```python
from build123d import *

# Parameters (mm, degrees)
SKETCH1_R           = 4.5
SKETCH1_R_2         = 5
BOSS_EXTRUDE2_DEPTH = 3


with BuildPart() as part:
    # Sketch1 → Boss-Extrude2 (new body)
    with BuildSketch(Plane.XY):
        with BuildLine():
            Line((400, 6), (0, 6))
            ThreePointArc((0, 6), (-6, 0), (0, -6))
            Line((0, -6), (95, -6))
            Line((95, -6), (95, -35))
            ThreePointArc((95, -35), (100, -40), (105, -35))
            Line((105, -35), (105, -6))
            Line((105, -6), (155, -6))
            Line((155, -6), (155, -35))
            ThreePointArc((155, -35), (160, -40), (165, -35))
            Line((165, -35), (165, -6))
            Line((165, -6), (215, -6))
            Line((215, -6), (215, -35))
            ThreePointArc((215, -35), (220, -40), (225, -35))
            Line((225, -35), (225, -6))
            Line((225, -6), (275, -6))
            Line((275, -6), (275, -35))
            ThreePointArc((275, -35), (280, -40), (285, -35))
            Line((285, -35), (285, -6))
            Line((285, -6), (400, -6))
            ThreePointArc((400, -6), (406, 0), (400, 6))
        make_face()
        Circle(SKETCH1_R, mode=Mode.SUBTRACT)
        with Locations((400, 0)):
            Circle(SKETCH1_R_2, mode=Mode.SUBTRACT)
        with Locations((100, -35)):
            Circle(SKETCH1_R, mode=Mode.SUBTRACT)
        with Locations((280, -35)):
            Circle(SKETCH1_R, mode=Mode.SUBTRACT)
        with Locations((160, -35)):
            Circle(SKETCH1_R, mode=Mode.SUBTRACT)
        with Locations((220, -35)):
            Circle(SKETCH1_R, mode=Mode.SUBTRACT)
    extrude(amount=BOSS_EXTRUDE2_DEPTH)


solid = part.part
```
Work out the finished part from the listing and answer in its coordinate system (mm). Coordinates: 2 decimals unless noted, no trailing zeros. Order: outer loops, then holes, each group sorted by start corner. A loop starts at its lowest first (then second) coordinate and runs counter-clockwise, first axis right, second up. Notation, with made-up numbers: M 13.5,-11 L 41.5,-11 A19 cw 41.5,6 Z; hole C 83,36.5 d8. An arc over 180 degrees is marked long. Use CSV: the item, a comma, the result in double quotes.
1) Consider line 1 (X direction, y = -23, z = 1.25); line 2 (Y direction, x = 160, z = 1.8); line 3 (Y direction, x = 400, z = 0.85). Determine where each line is inside the solid, lowest interval first. Write a range as [from, to].
Worked out:
line 1,"x = [95, 105], [155, 165], [215, 225], [275, 285]"
line 2,"y = [-40, -39.5], [-30.5, 6]"
line 3,"y = [-6, -5], [5, 6]"
2) Section D-D on x = 100 is taken. Write down the section's boundary in (y, z).
Worked out:
outline,"M -40,0 L -39.5,0 L -39.5,3 L -40,3 Z; M -30.5,0 L 6,0 L 6,3 L -30.5,3 Z"
3) Section A-A on y = -19.5 is taken. Write down the section's boundary in (x, z).
Worked out:
outline,"M 95,0 L 105,0 L 105,3 L 95,3 Z; M 155,0 L 165,0 L 165,3 L 155,3 Z; M 215,0 L 225,0 L 225,3 L 215,3 Z; M 275,0 L 285,0 L 285,3 L 275,3 Z"
4) Section B-B on y = 0 is taken. Write down the section's boundary in (x, z).
Worked out:
outline,"M -6,0 L -4.5,0 L -4.5,3 L -6,3 Z; M 4.5,0 L 395,0 L 395,3 L 4.5,3 Z; M 405,0 L 406,0 L 406,3 L 405,3 Z"
5) Flat-ended cylindrical pins translate along their axes: pin 1 Ø1.5 at (y, z) = (-18.5, 2) entering from -X; pin 2 Ø1.5 at (y, z) = (-17.5, 1.5) entering from +X; pin 3 Ø1.5 at (x, z) = (65, 2) entering from -Y. Find the tip coordinate at first contact, or state that the pin passes through.
Worked out:
pin 1,"stops at x = 95"
pin 2,"stops at x = 285"
pin 3,"stops at y = -6"
6) Determine the mould class of faces 1 (the face through (224.16, -36.72, 1.48)), 2 (the face through (-0.59, 4.46, 1.48)), 3 (the face through (199, -2, 0)) for opening direction X: released by +X, released by -X, zero draft, split by the parting line, or undercut.
Worked out:
face 1,"undercut"
face 2,"undercut"
face 3,"zero draft"
7) Section C-C on z = 1.1 is taken. Write down the section's boundary in (x, y), plus the area to 3 significant figures.
Worked out:
outline,"M 0,-6 L 95,-6 L 95,-35 A5 ccw 105,-35 L 105,-6 L 155,-6 L 155,-35 A5 ccw 165,-35 L 165,-6 L 215,-6 L 215,-35 A5 ccw 225,-35 L 225,-6 L 275,-6 L 275,-35 A5 ccw 285,-35 L 285,-6 L 400,-6 A6 ccw 400,6 L 0,6 A6 ccw Z; hole C 0,0 d9; hole C 100,-35 d9; hole C 160,-35 d9; hole C 220,-35 d9; hole C 280,-35 d9; hole C 400,0 d10"
area,"5,830 mm^2"
